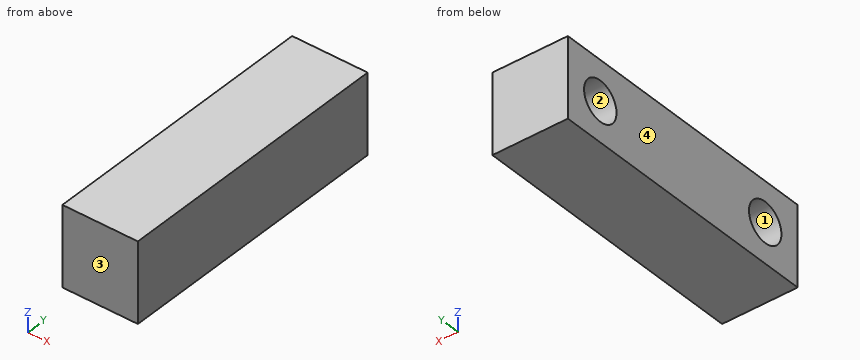
Autodesk Inventor part; units mm, degrees
ref_plane "YZ Plane" through (0, 0, 0) normal (1, 0, 0) x (0, 1, 0)
ref_plane "XZ Plane" through (0, 0, 0) normal (0, 1, 0) x (-1, 0, 0)
ref_plane "XY Plane" through (0, 0, 0) normal (0, 0, 1) x (1, 0, 0)
sketch "Sketch1" plane through (0, 0, 0) normal (0, 0, 1) x (1, 0, 0)
  line L0 (6, -22.5) -> (-6, -22.5)
  line L1 (-6, -22.5) -> (-6, 22.5)
  line L2 (-6, 22.5) -> (6, 22.5)
  line L3 (6, 22.5) -> (6, -22.5)
  line L4 (6, -22.5) -> (-6, 22.5) construction
  line L5 (-6, -22.5) -> (6, 22.5) construction
  line L6 (-5.1503, -35.0501) -> (13.5409, -35.0501)
  point P0 (0, 0)
  point P1 (4.1953, 105.9109)
  point P2 (0, 0)
  point P3 (11.236, -97.2891)
  point P4 (-6, 0)
  dimension "d0" = 12
  dimension "d1" = 45
  dimension "d2" = 57.55
extrude "Extrusion1" add sketch "Sketch1" along normal blind 12.7
sketch "Sketch3" plane through (-6, -22.5, 0) normal (-1, 0, 0) x (0, 0, 1)
  circle A0 centre (6.35, 38.65) radius 3.175
  line L0 (12.7, 45) -> (12.7, 0)
  line L1 (0, 45) -> (12.7, 45)
  circle A1 centre (6.35, 6.35) radius 3.175
  line L2 (0, 0) -> (12.7, 0)
  point P0 (0, 22.5)
  point P1 (6.35, 45)
  dimension "d10" = 6.35
  dimension "d11" = 6.35
  dimension "d12" = 6.35
  dimension "d13" = 6.35
  dimension "d14" = 6.35
  dimension "d15" = 6.35
extrude "Extrusion3" cut sketch "Sketch3" against normal blind 6.35
properties part number "EndCap"
Work out the finished part from the listing and answer in its coordinate system (mm). Face numbers are marked on the shaded views. Give positions to 0.01 mm unless a question says otherwise; leave off trailing zeros. Loops run counter-clockwise (first coordinate to the right, second up) from the corner with the lowest first, then second, coordinate; pieces in that order, holes last. Notation, with made-up numbers: (-29.75, 37) -> (-3.75, 37) arc R20 ccw to (-3.75, 46) -> close; hole circle Ø10 at (73.5, 60). An arc over 180 degrees is marked (long way). Use CSV: the item, a comma, the result in double quotes.
1. The mould has two halves that part along Y. Classify the marked faces 1, 2, 3 and 4: +Y half, -Y half, draft (parallel to the pull), parting line (faces both ways), or undercut.
Found:
face 1,"undercut"
face 2,"undercut"
face 3,"-Y half"
face 4,"draft"
2. The part is cut by section A-A (x = -0.25). Write down the section's boundary in (y, z) (3 decimals), then the cut area to 3 significant figures.
Found:
outline,"(-22.5, 0) -> (22.5, 0) -> (22.5, 12.7) -> (-22.5, 12.7) -> close; hole circle Ø6.35 at (-16.15, 6.35); hole circle Ø6.35 at (16.15, 6.35)"
area,"508 mm^2"
3. The part is cut by section B-B (y = -16.15). Write down the section's boundary in (x, z) (3 decimals).
Found:
outline,"(-6, 0) -> (6, 0) -> (6, 12.7) -> (-6, 12.7) -> (-6, 9.525) -> (0.35, 9.525) -> (0.35, 3.175) -> (-6, 3.175) -> close"
4. Straight lines are drawn through the part: line 1 (Y direction, x = -3.75, z = 6.35) (3 decimals); line 2 (X direction, y = 17, z = 9). For each, find the intervals that lie inside material, in ascending order.
Found:
line 1,"-22.5 to -19.325, -12.975 to 12.975, 19.325 to 22.5"
line 2,"0.35 to 6"
5. Flat-ended cylindrical pins translate along their axes: pin 1 Ø1.9 at (y, z) = (-17.5, 6.5) entering from -X; pin 2 Ø7 at (y, z) = (16, 7.5) entering from -X. Find the tip coordinate at first contact, or state that the pin passes through.
Found:
pin 1,"x = 0.35"
pin 2,"x = -6"
6. The part is cut by section D-D (z = 9). Write down the section's boundary in (x, y).
Found:
outline,"(-6, -22.5) -> (6, -22.5) -> (6, 22.5) -> (-6, 22.5) -> (-6, 17.9) -> (0.35, 17.9) -> (0.35, 14.4) -> (-6, 14.4) -> (-6, -14.4) -> (0.35, -14.4) -> (0.35, -17.9) -> (-6, -17.9) -> close"
7. The part is cut by section C-C (z = 6.35). Write down the section's boundary in (x, y) (3 decimals), then the cut area to 3 significant figures.
Found:
outline,"(-6, -22.5) -> (6, -22.5) -> (6, 22.5) -> (-6, 22.5) -> (-6, 19.325) -> (0.35, 19.325) -> (0.35, 12.975) -> (-6, 12.975) -> (-6, -12.975) -> (0.35, -12.975) -> (0.35, -19.325) -> (-6, -19.325) -> close"
area,"459 mm^2"
